from build123d import *

# Parameters (mm, degrees)
F0_W     = 404
F0_H     = 145
F2_DEPTH = 3
F3_D     = 3.3
F3_DEPTH = 8.6
F3_TIP   = 0.9914200214
F1_R     = 1.5
F1_R_2   = 15
F1_R_3   = 1.75
F1_W     = 53.5
F1_H     = 13
F1_R_4   = 2.5
F4_DEPTH = 25


with BuildPart() as f2:
    # F0 (on Top) → F2 (new body)
    with BuildSketch(Plane.XY):
        with Locations((-14.1859020234, -7.6260944492)):
            Rectangle(F0_W, F0_H)
    extrude(amount=-F2_DEPTH)

    # F3
    with Locations(Plane.XY):
        with Locations((118.573140085, 24.8739055508), (158.573140085, 24.8739055508), (93.573140085, 24.8739055508), (53.573140085, 24.8739055508), (53.573140085, -40.1260944492), (93.573140085, -40.1260944492), (118.573140085, -40.1260944492), (158.573140085, -40.1260944492), (28.573140085, -40.1260944492), (-11.426859915, -40.1260944492), (-11.426859915, 24.8739055508), (28.573140085, 24.8739055508), (-35.926859915, 24.8739055508), (-80.926859915, 24.8739055508), (-80.926859915, -40.1260944492), (-35.926859915, -40.1260944492)):
            Hole(F3_D / 2, depth=F3_DEPTH)
            with Locations((0, 0, -(F3_DEPTH + F3_TIP / 2))):  # 118° drill point
                Cone(0, F3_D / 2, F3_TIP, mode=Mode.SUBTRACT)

    # F1 (on Top) → F4 (cut)
    with BuildSketch(Plane.XY):
        with BuildLine():
            Line((126.323140085, 12.4739055508), (150.823140085, 12.4739055508))
            ThreePointArc((150.823140085, 12.4739055508), (153.6515672098, 13.645478426), (154.823140085, 16.4739055508))
            Line((154.823140085, 16.4739055508), (154.823140085, 33.2739055508))
            ThreePointArc((154.823140085, 33.2739055508), (153.6515672098, 36.1023326755), (150.823140085, 37.2739055508))
            Line((150.823140085, 37.2739055508), (126.323140085, 37.2739055508))
            ThreePointArc((126.323140085, 37.2739055508), (123.4947129603, 36.1023326755), (122.323140085, 33.2739055508))
            Line((122.323140085, 33.2739055508), (122.323140085, 16.4739055508))
            ThreePointArc((122.323140085, 16.4739055508), (123.4947129603, 13.645478426), (126.323140085, 12.4739055508))
        make_face()
        with Locations((158.573140085, 24.8739055508)):
            Circle(F1_R)
        with Locations((118.573140085, 24.8739055508)):
            Circle(F1_R)
        with BuildLine():
            Line((-72.226859915, 10.1239055508), (-44.626859915, 10.1239055508))
            ThreePointArc((-44.626859915, 10.1239055508), (-41.091326009, 11.5883716448), (-39.626859915, 15.1239055508))
            Line((-39.626859915, 15.1239055508), (-39.626859915, 34.6239055508))
            ThreePointArc((-39.626859915, 34.6239055508), (-41.091326009, 38.1594394567), (-44.626859915, 39.6239055508))
            Line((-44.626859915, 39.6239055508), (-72.226859915, 39.6239055508))
            ThreePointArc((-72.226859915, 39.6239055508), (-75.7623938209, 38.1594394567), (-77.226859915, 34.6239055508))
            Line((-77.226859915, 34.6239055508), (-77.226859915, 15.1239055508))
            ThreePointArc((-77.226859915, 15.1239055508), (-75.7623938209, 11.5883716448), (-72.226859915, 10.1239055508))
        make_face()
        with Locations((-35.926859915, 24.8739055508)):
            Circle(F1_R)
        with Locations((-80.926859915, 24.8739055508)):
            Circle(F1_R)
        with BuildLine():
            Line((122.323140085, -31.7260944492), (122.323140085, -48.5260944492))
            ThreePointArc((122.323140085, -48.5260944492), (123.4947129603, -51.354521574), (126.323140085, -52.5260944492))
            Line((126.323140085, -52.5260944492), (150.823140085, -52.5260944492))
            ThreePointArc((150.823140085, -52.5260944492), (153.6515672098, -51.354521574), (154.823140085, -48.5260944492))
            Line((154.823140085, -48.5260944492), (154.823140085, -31.7260944492))
            ThreePointArc((154.823140085, -31.7260944492), (153.6515672098, -28.8976673245), (150.823140085, -27.7260944492))
            Line((150.823140085, -27.7260944492), (126.323140085, -27.7260944492))
            ThreePointArc((126.323140085, -27.7260944492), (123.4947129603, -28.8976673245), (122.323140085, -31.7260944492))
        make_face()
        with Locations((158.573140085, -40.1260944492)):
            Circle(F1_R)
        with Locations((118.573140085, -40.1260944492)):
            Circle(F1_R)
        with BuildLine():
            Line((57.323140085, 33.2739055508), (57.323140085, 16.4739055508))
            ThreePointArc((57.323140085, 16.4739055508), (58.4947129603, 13.645478426), (61.323140085, 12.4739055508))
            Line((61.323140085, 12.4739055508), (85.823140085, 12.4739055508))
            ThreePointArc((85.823140085, 12.4739055508), (88.6515672098, 13.645478426), (89.823140085, 16.4739055508))
            Line((89.823140085, 16.4739055508), (89.823140085, 33.2739055508))
            ThreePointArc((89.823140085, 33.2739055508), (88.6515672098, 36.1023326755), (85.823140085, 37.2739055508))
            Line((85.823140085, 37.2739055508), (61.323140085, 37.2739055508))
            ThreePointArc((61.323140085, 37.2739055508), (58.4947129603, 36.1023326755), (57.323140085, 33.2739055508))
        make_face()
        with Locations((93.573140085, 24.8739055508)):
            Circle(F1_R)
        with Locations((53.573140085, 24.8739055508)):
            Circle(F1_R)
        with BuildLine():
            Line((57.323140085, -31.7260944492), (57.323140085, -48.5260944492))
            ThreePointArc((57.323140085, -48.5260944492), (58.4947129603, -51.354521574), (61.323140085, -52.5260944492))
            Line((61.323140085, -52.5260944492), (85.823140085, -52.5260944492))
            ThreePointArc((85.823140085, -52.5260944492), (88.6515672098, -51.354521574), (89.823140085, -48.5260944492))
            Line((89.823140085, -48.5260944492), (89.823140085, -31.7260944492))
            ThreePointArc((89.823140085, -31.7260944492), (88.6515672098, -28.8976673245), (85.823140085, -27.7260944492))
            Line((85.823140085, -27.7260944492), (61.323140085, -27.7260944492))
            ThreePointArc((61.323140085, -27.7260944492), (58.4947129603, -28.8976673245), (57.323140085, -31.7260944492))
        make_face()
        with Locations((93.573140085, -40.1260944492)):
            Circle(F1_R)
        with Locations((53.573140085, -40.1260944492)):
            Circle(F1_R)
        with BuildLine():
            Line((-7.676859915, 33.2739055508), (-7.676859915, 16.4739055508))
            ThreePointArc((-7.676859915, 16.4739055508), (-6.5052870397, 13.645478426), (-3.676859915, 12.4739055508))
            Line((-3.676859915, 12.4739055508), (20.823140085, 12.4739055508))
            ThreePointArc((20.823140085, 12.4739055508), (23.6515672098, 13.645478426), (24.823140085, 16.4739055508))
            Line((24.823140085, 16.4739055508), (24.823140085, 33.2739055508))
            ThreePointArc((24.823140085, 33.2739055508), (23.6515672098, 36.1023326755), (20.823140085, 37.2739055508))
            Line((20.823140085, 37.2739055508), (-3.676859915, 37.2739055508))
            ThreePointArc((-3.676859915, 37.2739055508), (-6.5052870397, 36.1023326755), (-7.676859915, 33.2739055508))
        make_face()
        with Locations((28.573140085, 24.8739055508)):
            Circle(F1_R)
        with Locations((-11.426859915, 24.8739055508)):
            Circle(F1_R)
        with BuildLine():
            Line((-7.676859915, -31.7260944492), (-7.676859915, -48.5260944492))
            ThreePointArc((-7.676859915, -48.5260944492), (-6.5052870397, -51.354521574), (-3.676859915, -52.5260944492))
            Line((-3.676859915, -52.5260944492), (20.823140085, -52.5260944492))
            ThreePointArc((20.823140085, -52.5260944492), (23.6515672098, -51.354521574), (24.823140085, -48.5260944492))
            Line((24.823140085, -48.5260944492), (24.823140085, -31.7260944492))
            ThreePointArc((24.823140085, -31.7260944492), (23.6515672098, -28.8976673245), (20.823140085, -27.7260944492))
            Line((20.823140085, -27.7260944492), (-3.676859915, -27.7260944492))
            ThreePointArc((-3.676859915, -27.7260944492), (-6.5052870397, -28.8976673245), (-7.676859915, -31.7260944492))
        make_face()
        with Locations((28.573140085, -40.1260944492)):
            Circle(F1_R)
        with Locations((-11.426859915, -40.1260944492)):
            Circle(F1_R)
        with BuildLine():
            Line((-77.226859915, -30.3760944492), (-77.226859915, -49.8760944492))
            ThreePointArc((-77.226859915, -49.8760944492), (-75.7623938209, -53.4116283552), (-72.226859915, -54.8760944492))
            Line((-72.226859915, -54.8760944492), (-44.626859915, -54.8760944492))
            ThreePointArc((-44.626859915, -54.8760944492), (-41.091326009, -53.4116283552), (-39.626859915, -49.8760944492))
            Line((-39.626859915, -49.8760944492), (-39.626859915, -30.3760944492))
            ThreePointArc((-39.626859915, -30.3760944492), (-41.091326009, -26.8405605433), (-44.626859915, -25.3760944492))
            Line((-44.626859915, -25.3760944492), (-72.226859915, -25.3760944492))
            ThreePointArc((-72.226859915, -25.3760944492), (-75.7623938209, -26.8405605433), (-77.226859915, -30.3760944492))
        make_face()
        with Locations((-35.926859915, -40.1260944492)):
            Circle(F1_R)
        with Locations((-80.926859915, -40.1260944492)):
            Circle(F1_R)
        with Locations((-181.676859915, -40.1260944492)):
            Circle(F1_R_2)
        with Locations((-169.176859915, -55.1260944492)):
            Circle(F1_R_3)
        with Locations((-194.176859915, -25.1260944492)):
            Circle(F1_R_3)
        with Locations((-181.676859915, 24.8739055508)):
            Rectangle(F1_W, F1_H)
        with Locations((-205.6832462549, 57.1586787701)):
            Circle(F1_R_4)
        with BuildLine():
            Line((-128.976859915, -35.8176724643), (-128.976859915, -44.4345164341))
            ThreePointArc((-128.976859915, -44.4345164341), (-122.176859915, -48.1760944492), (-115.376859915, -44.4345164341))
            Line((-115.376859915, -44.4345164341), (-115.376859915, -35.8176724643))
            ThreePointArc((-115.376859915, -35.8176724643), (-122.176859915, -32.0760944492), (-128.976859915, -35.8176724643))
        make_face()
        with Locations((-122.176859915, 24.8739055508)):
            Rectangle(F1_W, F1_H)
    extrude(amount=-F4_DEPTH, mode=Mode.SUBTRACT)


solid = f2.part
Here's how the part is built. I have some questions about the finished solid (model axes, mm). Round coordinates to 2 decimals unless told otherwise and drop trailing zeros. Write each loop counter-clockwise with the first axis right and the second up, starting at its lowest first coordinate (ties: lowest second). Pieces come first, ordered by that corner, then holes.
1. Will this pin go through, and if not, where does the flat tip stop? pin 1 Ø3 at (x, y) = (-205.68, 57.16) entering from +Z.
2. Suppose I cut it at A-A (x = 138.5). List the corners of the cut face in (y, z) for me.
3. Suppose I cut it at C-C (z = -1.9). State how many separate pieces and enclosed holes the cut face has, and give its area (3 significant figures).
4. Suppose I cut it at B-B (x = -60). List the corners of the cut face in (y, z) for me, and give its area (3 significant figures).
5. I need wall thicknesses on L1, parallel to Y at x = 71, z = -2.2; L2, parallel to Y at x = -62.5, z = -2.75; L3, parallel to Y at x = -159, z = -1.15. Which ranges of each line are inside material? Lowest first, please.
6. If we mould it in two halves opening along X, with no side actions, what happens to faces 1 (the flat face through (-17, -7, -3)), 2 (the cylindrical face through (-167.37, -35.62, -1.48))? For each: released by +X, released by -X, zero draft, split by the parting line, or undercut.
Answer sheet:
1. pin 1: passes through
2. outline: (-80.13, -3) - (-52.53, -3) - (-52.53, 0) - (-80.13, 0) - close; (-27.73, -3) - (12.47, -3) - (12.47, 0) - (-27.73, 0) - close; (37.27, -3) - (64.87, -3) - (64.87, 0) - (37.27, 0) - close
3. separate pieces: 1
3. enclosed holes: 31
3. area: 49,200 mm2
4. outline: (-80.13, -3) - (-54.88, -3) - (-54.88, 0) - (-80.13, 0) - close; (-25.38, -3) - (10.12, -3) - (10.12, 0) - (-25.38, 0) - close; (39.62, -3) - (64.87, -3) - (64.87, 0) - (39.62, 0) - close
4. area: 258 mm2
5. L1: y = -80.13 to -52.53, -27.73 to 12.47, 37.27 to 64.87
5. L2: y = -80.13 to -54.88, -25.38 to 10.12, 39.62 to 64.87
5. L3: y = -80.13 to 18.37, 31.37 to 64.87
6. face 1: zero draft
6. face 2: undercut
